Part model, mm, in its own coordinate system. Coordinates: 2 decimals unless noted, no trailing zeros. Write each loop counter-clockwise with the first axis right and the second up, starting at its lowest first coordinate (ties: lowest second). Pieces come first, ordered by that corner, then holes. Notation, with made-up numbers: M 82,50 L 126,50 A13 cw 126,60 Z; hole C 37.5,56 d11. An arc over 180 degrees is marked long. Use a Markdown table: item, result. Add a question column.
Q1. Slice it at C-C on z = 97.5. Write the cut outline in (x, y) (3 decimals), then the cut area to 3 significant figures.
Q2. Wall check: L1, parallel to X at y = 3, z = -135; L2, parallel to X at y = -4.5, z = -38. Give the ranges that are in metal, low to high. Write a range as from..to.
Q3. Slice it at A-A on x = 0. Write the cut outline in (y, z), then the cut area to 3 significant figures.
from build123d import *

# Parameters (mm, degrees)
BOSS_EXTRUDE1_DEPTH          = 152.4
BOSS_EXTRUDE1_DEPTH_BACK     = 152.4
F_3_8_0_375_DIAMETER_HOLE1_D = 9.525
F_3_8_0_375_DIAMETER_HOLE2_D = 9.525


with BuildPart() as part:
    # Sketch4 → Boss-Extrude1 (new, two sides: drawn at the far end of the back side and taken through both)
    with BuildSketch(Plane.XY.offset(-BOSS_EXTRUDE1_DEPTH_BACK)):
        with BuildLine():
            Line((6.35, -5.715), (6.35, 5.715))
            ThreePointArc((6.35, 5.715), (6.164012806, 6.164012806), (5.715, 6.35))
            Line((5.715, 6.35), (-5.715, 6.35))
            ThreePointArc((-5.715, 6.35), (-6.164012806, 6.164012806), (-6.35, 5.715))
            Line((-6.35, 5.715), (-6.35, -5.715))
            ThreePointArc((-6.35, -5.715), (-6.164012806, -6.164012806), (-5.715, -6.35))
            Line((-5.715, -6.35), (5.715, -6.35))
            ThreePointArc((5.715, -6.35), (6.164012806, -6.164012806), (6.35, -5.715))
        make_face()
        with BuildLine():
            Line((4.699, 4.2291), (4.699, -4.2291))
            ThreePointArc((4.699, -4.2291), (4.561369476, -4.561369476), (4.2291, -4.699))
            Line((4.2291, -4.699), (-4.2291, -4.699))
            ThreePointArc((-4.2291, -4.699), (-4.561369476, -4.561369476), (-4.699, -4.2291))
            Line((-4.699, -4.2291), (-4.699, 4.2291))
            ThreePointArc((-4.699, 4.2291), (-4.561369476, 4.561369476), (-4.2291, 4.699))
            Line((-4.2291, 4.699), (4.2291, 4.699))
            ThreePointArc((4.2291, 4.699), (4.561369476, 4.561369476), (4.699, 4.2291))
        make_face(mode=Mode.SUBTRACT)
    extrude(amount=BOSS_EXTRUDE1_DEPTH + BOSS_EXTRUDE1_DEPTH_BACK)

    # 3/8 (0.375) Diameter Hole1 (through all)
    with Locations(Plane(origin=(0, 6.35, 0), x_dir=(1, 0, 0), z_dir=(0, 1, 0))):
        with Locations((0, 88.088749974)):
            Hole(F_3_8_0_375_DIAMETER_HOLE1_D / 2)

    # 3/8 (0.375) Diameter Hole2 (through all)
    with Locations(Plane(origin=(0, 6.35, 0), x_dir=(1, 0, 0), z_dir=(0, 1, 0))):
        with Locations((0, 18.166595951)):
            Hole(F_3_8_0_375_DIAMETER_HOLE2_D / 2)


solid = part.part
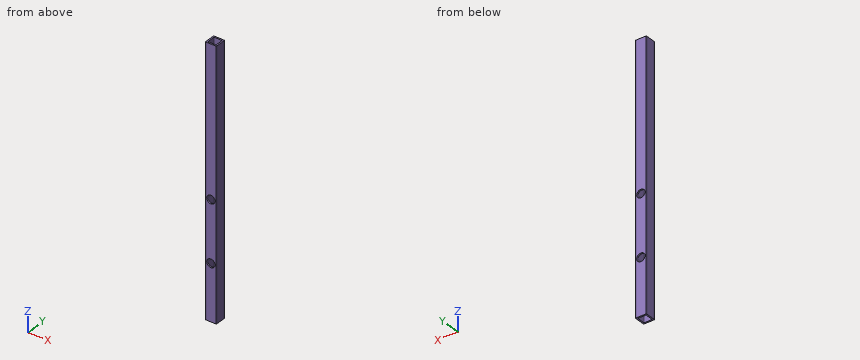
Recorded:
| question | item | result |
|---|---|---|
| 1 | outline | M -6.35,-5.715 A0.635 ccw -5.715,-6.35 L 5.715,-6.35 A0.635 ccw 6.35,-5.715 L 6.35,5.715 A0.635 ccw 5.715,6.35 L -5.715,6.35 A0.635 ccw -6.35,5.715 Z; hole M -4.699,-4.229 A0.47 ccw -4.229,-4.699 L 4.229,-4.699 A0.47 ccw 4.699,-4.229 L 4.699,4.229 A0.47 ccw 4.229,4.699 L -4.229,4.699 A0.47 ccw -4.699,4.229 Z |
| 1 | area | 72.8 mm² |
| 2 | L1 | -6.35..-4.7, 4.7..6.35 |
| 2 | L2 | -6.35..-4.61, 4.61..6.35 |
| 3 | outline | M -6.35,-152.4 L -4.7,-152.4 L -4.7,-92.85 L -6.35,-92.85 Z; M -6.35,-83.33 L -4.7,-83.33 L -4.7,-22.93 L -6.35,-22.93 Z; M -6.35,-13.4 L -4.7,-13.4 L -4.7,152.4 L -6.35,152.4 Z; M 4.7,-152.4 L 6.35,-152.4 L 6.35,-92.85 L 4.7,-92.85 Z; M 4.7,-83.33 L 6.35,-83.33 L 6.35,-22.93 L 4.7,-22.93 Z; M 4.7,-13.4 L 6.35,-13.4 L 6.35,152.4 L 4.7,152.4 Z |
| 3 | area | 944 mm² |
